Model file for the job. Use its own axes, mm. Face numbers are marked on the shaded views. Give positions to 0.01 mm unless a question says otherwise; leave off trailing zeros. Loops run counter-clockwise (first coordinate to the right, second up) from the corner with the lowest first, then second, coordinate; pieces in that order, holes last. Notation, with made-up numbers: M 50.25,61.25 L 77.25,61.25 A20 cw 77.25,81.25 Z; hole C 1,35 d5. An arc over 180 degrees is marked long. Answer in a Markdown table with one row per item.
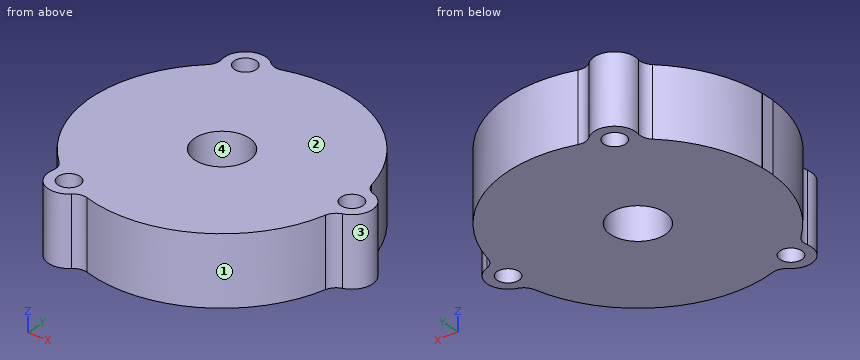
Autodesk Inventor part; units mm, degrees
ref_plane "Work Plane1" through (-44.1783, -54.1783, 25) normal (0, 0, -1) x (0.3122, 0.95, 0)
ref_plane "YZ Plane" through (0, 0, 0) normal (1, 0, 0) x (0, 1, 0)
ref_plane "XZ Plane" through (0, 0, 0) normal (0, 1, 0) x (-1, 0, 0)
sketch "Sketch1" plane through (0, 0, 0) normal (0, 0, 1) x (1, 0, 0)
  circle A0 centre (0, -10) radius 10
  circle A1 centre (47.5, -10) radius 4
  arc A2 (-13.75, -55.4663) -> (46.25, -20.8253) centre (0, -10) ccw
  arc A3 (49.6711, -17.1789) -> (46.25, -20.8253) centre (51.1184, -21.9648) ccw
  arc A4 (49.6711, -17.1789) -> (49.6711, -2.8211) centre (47.5, -10) ccw
  arc A5 (46.25, 0.8253) -> (49.6711, -2.8211) centre (51.1184, 1.9648) ccw
  arc A6 (46.25, 0.8253) -> (-13.75, 35.4663) centre (0, -10) ccw
  arc A7 (-18.6184, 36.6058) -> (-13.75, 35.4663) centre (-15.1974, 40.2523) ccw
  arc A8 (-18.6184, 36.6058) -> (-31.0526, 29.4269) centre (-23.75, 31.1362) ccw
  arc A9 (-32.5, 24.641) -> (-31.0526, 29.4269) centre (-35.9211, 28.2874) ccw
  arc A10 (-32.5, 24.641) -> (-47.4342, -7.5) centre (0, -10) ccw
  line L0 (-47.5, -7.5) -> (-47.4342, -7.5)
  line L1 (-47.5, -7.5) -> (-47.5, -12.5)
  line L2 (-47.4342, -12.5) -> (-47.5, -12.5)
  arc A11 (-47.4342, -12.5) -> (-32.5, -44.641) centre (0, -10) ccw
  arc A12 (-31.0526, -49.4269) -> (-32.5, -44.641) centre (-35.9211, -48.2874) ccw
  arc A13 (-31.0526, -49.4269) -> (-18.6184, -56.6058) centre (-23.75, -51.1362) ccw
  arc A14 (-13.75, -55.4663) -> (-18.6184, -56.6058) centre (-15.1974, -60.2523) ccw
  circle A15 centre (-23.75, 31.1362) radius 4
  circle A16 centre (-23.75, -51.1362) radius 4
  point P0 (0, 0)
ref_plane "Work Plane1" through (-44.1783, -54.1783, 25) normal (0, 0, -1) x (0.3122, 0.95, 0)
extrude "Extrusion1" add sketch "Sketch1" along normal up to surface (25 mm away)
properties part number "Motor Spacer"
Q1. Mould opens along Y. For the marked faces 1, 2, 3 and 4 say: released by +Y, released by -Y, zero draft, split by the parting line, or undercut.
Reported:
| item | result |
|---|---|
| face 1 | released by -Y |
| face 2 | zero draft |
| face 3 | split by the parting line |
| face 4 | undercut |
Q2. Saw through at C-C (z = 6). Give the cut face in (x, y).
Reported:
| item | result |
|---|---|
| outline | M -47.5,-12.5 L -47.43,-12.5 A47.5 ccw -32.5,-44.64 A5 cw -31.05,-49.43 A7.5 ccw -18.62,-56.61 A5 cw -13.75,-55.47 A47.5 ccw 46.25,-20.83 A5 cw 49.67,-17.18 A7.5 ccw 49.67,-2.82 A5 cw 46.25,0.83 A47.5 ccw -13.75,35.47 A5 cw -18.62,36.61 A7.5 ccw -31.05,29.43 A5 cw -32.5,24.64 A47.5 ccw -47.43,-7.5 L -47.5,-7.5 Z; hole C -23.75,-51.14 d8; hole C -23.75,31.14 d8; hole C 0,-10 d20; hole C 47.5,-10 d8 |
Q3. Saw through at B-B (x = 0). Give the cut face in (y, z), and give its area (4 significant figures).
Reported:
| item | result |
|---|---|
| outline | M -57.5,0 L -20,0 L -20,25 L -57.5,25 Z; M 0,0 L 37.5,0 L 37.5,25 L 0,25 Z |
| area | 1,875 mm² |
Q4. Drop flat-ended pins along their axis: pin 1 (12 mm diameter, centred on y = 8.5, z = 11.5, fed in from +X); pin 2 (2 mm diameter, centred on y = 24, z = 15, fed in from -X) (3 decimals); pin 3 (4 mm diameter, centred on y = -13, z = 16, fed in from +X). Give the stop position or say it passes through.
Reported:
| item | result |
|---|---|
| pin 1 | x = 45.83 |
| pin 2 | x = -34.165 |
| pin 3 | x = 54.93 |
Q5. Saw through at D-D (x = 47.5). Give the cut face in (y, z), and give its area (3 significant figures).
Reported:
| item | result |
|---|---|
| outline | M -18.51,0 L -14,0 L -14,25 L -18.51,25 Z; M -6,0 L -1.49,0 L -1.49,25 L -6,25 Z |
| area | 226 mm² |
Q6. Probe probe 1 along Y at (x, z) = (-23.75, 11); probe 2 along X at (y, z) = (-10.5, 8.75); probe 3 along Y at (x, z) = (0, 9). List the from-to ranges inside material, lowest first.
Reported:
| item | result |
|---|---|
| probe 1 | -58.64 to -55.14, -47.14 to 27.14, 35.14 to 38.64 |
| probe 2 | -47.5 to -9.99, 9.99 to 43.53, 51.47 to 54.98 |
| probe 3 | -57.5 to -20, 0 to 37.5 |
Q7. Saw through at A-A (x = -23.75). Give the cut face in (y, z).
Reported:
| item | result |
|---|---|
| outline | M -58.64,0 L -55.14,0 L -55.14,25 L -58.64,25 Z; M -47.14,0 L 27.14,0 L 27.14,25 L -47.14,25 Z; M 35.14,0 L 38.64,0 L 38.64,25 L 35.14,25 Z |
